Work out the finished part from the listing and answer in its coordinate system (mm). Face numbers are marked on the shaded views. A direction names the side the tool comes from. Round coordinates to 2 decimals unless told otherwise and drop trailing zeros. Order: outer loops, then holes, each group sorted by start corner. A loop starts at its lowest first (then second) coordinate and runs counter-clockwise, first axis right, second up.
Autodesk Inventor part; units mm, degrees
ref_plane "YZ Plane" through (0, 0, 0) normal (1, 0, 0) x (0, 1, 0)
ref_plane "XZ Plane" through (0, 0, 0) normal (0, 1, 0) x (-1, 0, 0)
ref_plane "XY Plane" through (0, 0, 0) normal (0, 0, 1) x (1, 0, 0)
sketch "Boceto2" plane through (0, 0, 0) normal (0, 0, 1) x (1, 0, 0)
  line L0 (-20, -10) -> (20, -10)
  line L1 (20, -10) -> (20, 10)
  line L2 (20, 10) -> (-20, 10)
  line L3 (-20, 10) -> (-20, -10)
  line L4 (-20, -10) -> (20, 10) construction
  line L5 (20, -10) -> (-20, 10) construction
  line L6 (-20, 10) -> (-10, 20)
  line L7 (10, 20) -> (20, 10)
  line L8 (-10, 20) -> (10, 20)
  point P0 (0, 0)
  dimension "d0" = 20
  dimension "d1" = 40
  dimension "d2" = 10
  dimension "d3" = 10
  dimension "d4" = 10
extrude "Extrusión1" add sketch "Boceto2" along normal blind 35
sketch "Boceto3" plane through (0, 0, 35) normal (0, 0, 1) x (1, 0, 0)
  circle A0 centre (0, 5) radius 10
  line L0 (-20, -10) -> (20, -10)
  point P0 (0, 0)
  dimension "d7" = 20
  dimension "d8" = 15
hole "Agujero1" at (0, 5, 35) direction (0, 0, -1) diameter 21 depth 35 tip angle 118
sketch "Boceto4" plane through (-20, -10, 0) normal (0, -1, 0) x (1, 0, 0)
  line L0 (5, 6) -> (35, 6)
  line L1 (35, 6) -> (35, 29)
  line L2 (35, 29) -> (5, 29)
  line L3 (5, 29) -> (5, 6)
  line L4 (5, 6) -> (35, 29) construction
  line L5 (35, 6) -> (5, 29) construction
  line L6 (40, 0) -> (40, 35)
  line L7 (30, 0) -> (30, 35)
  line L8 (0, 0) -> (0, 35)
  line L9 (0, 35) -> (40, 35)
  line L10 (0, 0) -> (40, 0)
  point P0 (20, 0)
  point P1 (20, 17.5)
  dimension "d16" = 23
  dimension "d17" = 5
  dimension "d18" = 10
  dimension "d19" = 5
  dimension "d20" = 30
  dimension "d30" = 17.5
  dimension "d31" = 35
hole "Agujero2" at (-15, -10, 29) at (15, -10, 29) at (15, -10, 6) at (-15, -10, 6) direction (0, 1, 0) diameter 3 depth 35 tip angle 118
sketch "Boceto6" plane through (-10, 20, 0) normal (0, 1, 0) x (1, 0, 0)
  line L0 (-5, -29) -> (25, -29)
  line L1 (25, -29) -> (25, -6)
  line L2 (25, -6) -> (-5, -6)
  line L3 (-5, -6) -> (-5, -29)
  line L4 (-5, -29) -> (25, -6) construction
  line L5 (25, -29) -> (-5, -6) construction
  line L6 (20, 0) -> (0, 0)
  point P0 (10, 0)
  point P1 (10, -17.5)
  dimension "d32" = 17.5
  dimension "d33" = 30
  dimension "d34" = 23
hole "Agujero3" at (15, 20, 29) at (-15, 20, 29) at (-15, 20, 6) at (15, 20, 6) direction (0, -1, 0) diameter 7 depth 10
properties part number "BracketLineal" material "Plástico ABS"
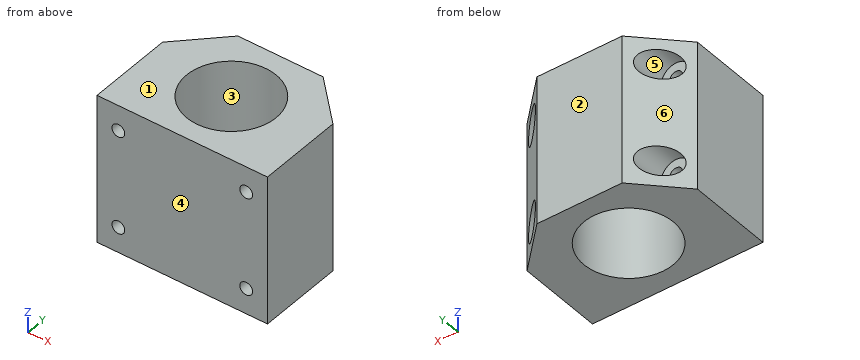
Item 1: For a pull along Y with two mould halves and no side action, classify the marked faces 1, 2, 3 and 4 as released by +Y, released by -Y, zero draft, split by the parting line, or undercut.
Item 2: Find the intervals of material crossed by line 1 along Z through (x, y) = (-15, 14.5); line 2 along Z through (x, y) = (-15, 6); line 3 along X through (y, z) = (5, 23), in increasing order.
Item 3: Find section D-D (z = 24.5). Write down the section's boundary in (x, y).
Item 4: A tool of negligible diameter and unlimited length cuts with its end or side. For the marked faces 5 and 6, from which of +Z, -Z, +X, -X, +Y, -Y can it reach the whole face along a straight path? Write none if from no direction.
Item 5: Find section B-B (x = 15). Write down the section's boundary in (y, z), plus the area to 3 significant figures.
Item 6: Find section C-C (y = 5). Write down the section's boundary in (x, z), plus the area to 3 significant figures.
Item 7: Given pin 1 (3.5 mm diameter, centred on x = -15, z = 30.5, fed in from +Y); pin 2 (1 mm diameter, centred on y = 11.5, z = 14.5, fed in from -X); pin 3 (8 mm diameter, centred on x = 0.5, y = 2.5, fed in from +Z); pin 4 (3.5 mm diameter, centred on x = 16.5, z = 4.5, fed in from +Y), each flat-ended and moving along its own axis, determine where each tip first touches the part or whether it passes through.
Item 8: Find section A-A (z = 29). Write down the section's boundary in (x, y).
Model answer:
1. face 1: zero draft
1. face 2: released by +Y
1. face 3: undercut
1. face 4: released by -Y
2. line 1: z = 0 to 2.5, 9.5 to 25.5, 32.5 to 35
2. line 2: z = 0 to 4.5, 7.5 to 27.5, 30.5 to 35
2. line 3: x = -20 to -10.5, 10.5 to 20
3. outline: (-20, -10) - (20, -10) - (20, 10) - (10, 20) - (-10, 20) - (-20, 10) - close; hole circle Ø21 at (0, 5)
4. face 5: +Y
4. face 6: +Z, -Z, -X, +Y
5. outline: (-10, 0) - (15, 0) - (15, 2.5) - (10, 2.5) - (10, 4.5) - (-10, 4.5) - close; (-10, 7.5) - (10, 7.5) - (10, 9.5) - (15, 9.5) - (15, 25.5) - (10, 25.5) - (10, 27.5) - (-10, 27.5) - close; (-10, 30.5) - (10, 30.5) - (10, 32.5) - (15, 32.5) - (15, 35) - (-10, 35) - close
5. area: 685 mm2
6. outline: (-20, 0) - (-10.5, 0) - (-10.5, 35) - (-20, 35) - close; (10.5, 0) - (20, 0) - (20, 35) - (10.5, 35) - close; hole circle Ø3 at (-15, 6); hole circle Ø3 at (-15, 29); hole circle Ø3 at (15, 6); hole circle Ø3 at (15, 29)
6. area: 637 mm2
7. pin 1: stops at y = 10
7. pin 2: stops at x = -19
7. pin 3: passes through
7. pin 4: stops at y = 13.68
8. outline: (-20, -10) - (-16.5, -10) - (-16.5, 10) - (-18.5, 10) - (-18.5, 11.5) - (-20, 10) - close; (-13.5, -10) - (13.5, -10) - (13.5, 10) - (11.5, 10) - (11.5, 18.5) - (10, 20) - (-10, 20) - (-11.5, 18.5) - (-11.5, 10) - (-13.5, 10) - close; (16.5, -10) - (20, -10) - (20, 10) - (18.5, 11.5) - (18.5, 10) - (16.5, 10) - close; hole circle Ø21 at (0, 5)
